The model under review builds one solid part; all positions refer to its coordinate system, in mm. Round coordinates to 2 decimals unless told otherwise and drop trailing zeros. Loops run counter-clockwise (first coordinate to the right, second up) from the corner with the lowest first, then second, coordinate; pieces in that order, holes last. Notation, with made-up numbers: M 36.25,30 L 95.25,30 A27 ccw 95.25,49 Z; hole C 60.25,2 d5. An arc over 180 degrees is marked long. Answer as a JSON object with one key per item and string values. Group by question number.
Item 1: Consider section A-A (z = 4.5). Give the boundary of the cut face in (x, y), and give its area (3 significant figures).
Item 2: Insertion check: P1, Ø5, axis at x = -45, y = -57, coming from the +Z side; P2, Ø2, axis at x = -39, z = 33, coming from the +Y side; P3, Ø12, axis at x = -20.5, z = 20, coming from the +Y side. Each pin has a flat end and moves straight along its axis. Give the tip position at first contact, or say it passes through.
Item 3: Consider section C-C (y = -27). Give the boundary of the cut face in (x, z), and give its area (3 significant figures).
Item 4: Consider section B-B (x = -48.5). Give the boundary of the cut face in (y, z), and give its area (3 significant figures).
Item 5: To check wall thickness, follow line 1 (X direction, y = -61, z = 6.5); line 2 (Y direction, x = -10, z = 29.5); line 3 (X direction, y = -19, z = 28). State the ranges of each line that lie inside material, in increasing order.
```python
from build123d import *

# Parameters (mm, degrees)
F0_W     = 152.4
F0_H     = 152.4
F1_DEPTH = 38.1
F2_SIZE  = 19.05
F3_SIZE  = 30.48


with BuildPart() as f1:
    # F0 (on Top) → F1 (new body)
    with BuildSketch(Plane.XY):
        Rectangle(F0_W, F0_H)
    extrude(amount=F1_DEPTH)

    # F2
    f2_edges = [f1.edges().sort_by_distance(p)[0] for p in [
        (-76.2, -76.2, 19.05),
        (76.2, -76.2, 19.05),
        (76.2, 76.2, 19.05),
        (-76.2, 76.2, 19.05),
    ]]
    chamfer(f2_edges, length=F2_SIZE)

    # F3
    f3_edges = [f1.edges().sort_by_distance(p)[0] for p in [
        (0, -76.2, 38.1),
        (-76.2, 0, 38.1),
        (0, 76.2, 38.1),
        (76.2, 0, 38.1),
        (66.675, -66.675, 38.1),
        (66.675, 66.675, 38.1),
        (-66.675, 66.675, 38.1),
        (-66.675, -66.675, 38.1),
    ]]
    chamfer(f3_edges, length=F3_SIZE)


solid = f1.part
```
Geometry results:
{
 "1": {"outline": "M -76.2,-57.15 L -57.15,-76.2 L 57.15,-76.2 L 76.2,-57.15 L 76.2,57.15 L 57.15,76.2 L -57.15,76.2 L -76.2,57.15 Z", "area": "22,500 mm^2"},
 "2": {"P1": "stops at z = 29.32", "P2": "stops at y = 51.82", "P3": "stops at y = 69.82"},
 "3": {"outline": "M -76.2,0 L 76.2,0 L 76.2,7.62 L 45.72,38.1 L -45.72,38.1 L -76.2,7.62 Z", "area": "4,880 mm^2"},
 "4": {"outline": "M -76.2,0 L 76.2,0 L 76.2,7.62 L 55.32,28.5 L 45.68,35.32 L -45.68,35.32 L -55.32,28.5 L -76.2,7.62 Z", "area": "4,600 mm^2"},
 "5": {"line 1": "x = -72.35 to 72.35", "line 2": "y = -54.32 to 54.32", "line 3": "x = -55.82 to 55.82"}
}
